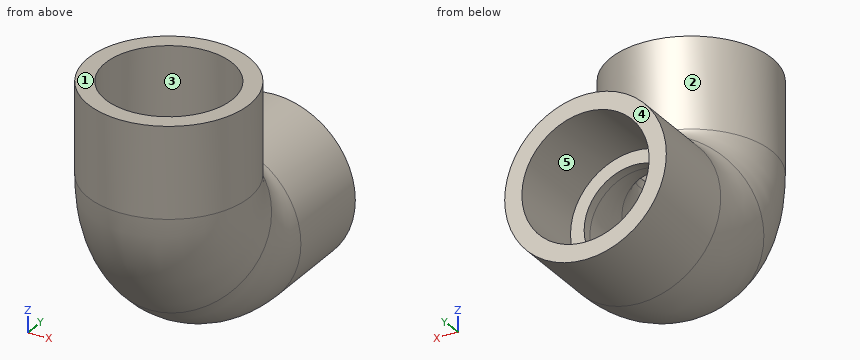
from build123d import *
from build123d import SkipClean  # not in build123d's __all__

# Parameters (mm, degrees)
F0_R        = 16.7005
F0_R_2      = 13.1191
F1_DEPTH    = 2.54
F0_R_3      = 21.209
F2_DEPTH    = 23.876
F2_FACE_R   = 21.209
F2_FACE_R_2 = 13.1191
F5_ANGLE    = 45


with BuildPart() as f1:
    # F0 (on Top) → F1 (new body)
    with BuildSketch(Plane.XY):
        Circle(F0_R)
        Circle(F0_R_2, mode=Mode.SUBTRACT)
    extrude(amount=F1_DEPTH)

    # F0 (on Top) → F2 (join)
    with BuildSketch(Plane.XY):
        Circle(F0_R_3)
        Circle(F0_R, mode=Mode.SUBTRACT)
    extrude(amount=F2_DEPTH)

    # F2_face (on face) → F5 (revolve)
    with BuildSketch(Plane(origin=(0, 0, 0), x_dir=(1, 0, 0), z_dir=(0, 0, -1))):
        Circle(F2_FACE_R)
        Circle(F2_FACE_R_2, mode=Mode.SUBTRACT)
    revolve(axis=Axis((12.7, 22.479, 0), (1, 0, 0)), revolution_arc=F5_ANGLE)

    # F6: F1 across face


with BuildPart() as f1_1:
    add(f1.part, clean=False)
    with SkipClean():  # cleaning this boolean's faces spoils the solid; the shape is the same uncleaned
        add(f1.part.mirror(Plane(origin=(0, 6.5839466657, -15.8950533343), x_dir=(-1, 0, 0), z_dir=(0, 0.7071067812, -0.7071067812))), clean=False)


solid = f1_1.part
The listing builds one solid part. Answer for the finished solid, in the listing's coordinates (mm). Face numbers are marked on the shaded views. A direction names the side the tool comes from. Give positions to 0.01 mm unless a question says otherwise; leave off trailing zeros. Order: outer loops, then holes, each group sorted by start corner. A loop starts at its lowest first (then second) coordinate and runs counter-clockwise, first axis right, second up. Notation, with made-up numbers: (22, -12) - (50, -12) arc R25 cw to (50, 18) - close; hole circle Ø6 at (3, 35.25). An arc over 180 degrees is marked (long way). One line per item, written item: value. Start each with the question number.
1) A cutting plane is placed at A-A on x = 0. Give the vertices of the cut face in (y, z) (1 decimal), then the cut area to 3 significant figures.
2) Find the intervals of material crossed by L1, parallel to Y at x = 0, z = 15; L2, parallel to Z at x = 0, y = 29.5; L3, parallel to Y at x = 0, z = 2.05, in increasing order.
3) A cutting plane is placed at B-B on y = 42. Give the vertices of the cut face in (x, z), then the cut area to 3 significant figures.
4) A cutting plane is placed at C-C on x = -14.5. Give the vertices of the cut face in (y, z) (3 decimals).
5) Given pin 1 Ø2 at (x, y) = (-2.5, 27.5) entering from +Z; pin 2 Ø6 at (y, z) = (35.5, -16) entering from -X; pin 3 Ø1.5 at (x, y) = (15, 33.5) entering from +Z; pin 4 Ø8 at (x, z) = (-9.5, -35.5) entering from +Y (3 decimals), each flat-ended and moving along its own axis, determine where each tip first touches the part or whether it passes through.
6) A tool of negligible diameter and unlimited length cuts with its end or side. For the marked faces 4 and 5, from which of +Z, -Z, +X, -X, +Y, -Y can it reach the whole face along a straight path? Write none if from no direction.
7) The mould has two halves that part along Y. Classify the marked faces 1, 2 and 3: released by +Y, released by -Y, zero draft, split by the parting line, or undercut.
Answer sheet:
1. outline: (-21.2, 0) arc R43.7 ccw to (22.5, -43.7) - (46.4, -43.7) - (46.4, -39.2) - (25, -39.2) - (25, -35.6) - (22.5, -35.6) arc R35.6 cw to (-13.1, 0) - (-13.1, 2.5) - (-16.7, 2.5) - (-16.7, 23.9) - (-21.2, 23.9) - close; (13.1, 0) arc R9.4 ccw to (22.5, -9.4) - (25, -9.4) - (25, -5.8) - (46.4, -5.8) - (46.4, -1.3) - (22.5, -1.3) arc R1.3 cw to (21.2, 0) - (21.2, 23.9) - (16.7, 23.9) - (16.7, 2.5) - (13.1, 2.5) - close
1. area: 1,040 mm2
2. L1: y = -21.21 to -16.7, 16.7 to 21.21
2. L2: z = -43.69 to -39.18, -5.78 to -1.27
2. L3: y = -21.21 to -13.12, 13.12 to 21.21
3. outline: circle Ø42.42 at (0, -22.48); hole circle Ø33.4 at (0, -22.48)
3. area: 537 mm2
4. outline: (-15.478, 0) arc R37.957 ccw to (22.479, -37.957) - (46.355, -37.957) - (46.355, -30.765) - (25.019, -30.765) - (25.019, -14.193) - (46.355, -14.193) - (46.355, -7.001) - (22.479, -7.001) arc R7.001 cw to (15.478, 0) - (15.478, 23.876) - (8.286, 23.876) - (8.286, 2.54) - (-8.286, 2.54) - (-8.286, 23.876) - (-15.478, 23.876) - close
5. pin 1: stops at z = -1.32
5. pin 2: stops at x = -20.92
5. pin 3: stops at z = -6.77
5. pin 4: stops at y = 46.355
6. face 4: +Z, -Z, +X, -X, +Y
6. face 5: +Y
7. face 1: zero draft
7. face 2: split by the parting line
7. face 3: undercut
